```python
from build123d import *

# Parameters (mm, degrees)
SKETCH_R     = 5.5
PAD_DEPTH    = 1
SKETCH001_R  = 4.1
PAD001_DEPTH = 3
SKETCH002_R  = 3.1
POCKET_DEPTH = 3.001


with BuildPart() as part:
    # Sketch → Pad (new body)
    with BuildSketch(Plane.XY):
        Circle(SKETCH_R)
    extrude(amount=PAD_DEPTH)

    # Sketch001 → Pad001 (join)
    with BuildSketch(Plane.XY):
        Circle(SKETCH001_R)
    extrude(amount=PAD001_DEPTH)

    # Sketch002 → Pocket (cut, through all)
    with BuildSketch(Plane.XY):
        Circle(SKETCH002_R)
    extrude(amount=POCKET_DEPTH, mode=Mode.SUBTRACT)


solid = part.part
```
Can you work these out from the model? Positions are in its coordinate system, mm. A direction names the side the tool comes from. Round coordinates to 2 decimals unless told otherwise and drop trailing zeros. Loops run counter-clockwise (first coordinate to the right, second up) from the corner with the lowest first, then second, coordinate; pieces in that order, holes last. Notation, with made-up numbers: M -28,1.5 L 9,1.5 A17 ccw 9,7.5 Z; hole C 84.5,55 d7. An arc over 180 degrees is marked long. Write item = value, one per line. Start each with the question number.
(1) Suppose I cut it at D-D on y = 3.5. Write out the boundary of the cut face in (x, z), plus the area to 3 significant figures.
(2) Which directions (+Z, -Z, +X, -X, +Y, -Y) give clear straight access to the entire face, cutting with the end or side of a thin tool? Please do faces 1 (the face through (-2, -4, 1)), 2 (the face through (-1.19, -5.37, 0.49)).
(3) I'm going to push flat-ended pins straight in: P1, Ø5, axis at x = 3, y = 4, coming from the +Z side; P2, Ø1.5, axis at y = -4, z = 2.5, coming from the -X side. Where does each tip first touch, or does it pass through?
(4) Suppose I cut it at A-A on y = 0. Write out the boundary of the cut face in (x, z), plus the area to 3 significant figures.
(5) Suppose I cut it at C-C on z = 1.7. Write out the boundary of the cut face in (x, y).
(6) I need wall thicknesses on line 1 along X through (y, z) = (0, 1.1); line 2 along Y through (x, z) = (0, 0.7). Which ranges of each line are inside material? Lowest first, please.
Answer block:
q1.outline = M -4.24,0 L 4.24,0 L 4.24,1 L 2.14,1 L 2.14,3 L -2.14,3 L -2.14,1 L -4.24,1 Z
q1.area = 17.0 mm²
q2.face_1 = +Z
q2.face_2 = +Z, -Z
q3.P1 = 3
q3.P2 = -2.5
q4.outline = M -5.5,0 L -3.1,0 L -3.1,3 L -4.1,3 L -4.1,1 L -5.5,1 Z; M 3.1,0 L 5.5,0 L 5.5,1 L 4.1,1 L 4.1,3 L 3.1,3 Z
q4.area = 8.80 mm²
q5.outline = C 0,0 d8.2; hole C 0,0 d6.2
q6.line_1 = -4.1 to -3.1, 3.1 to 4.1
q6.line_2 = -5.5 to -3.1, 3.1 to 5.5
